```python
from build123d import *

# Parameters (mm, degrees)
SKETCH2_R                   = 9.525
LID_HOLE_DEPTH              = 50.8
SKETCH5_R                   = 12.065
LID_MOUTHPIECE_DEPTH        = 13.97
SKETCH6_R                   = 9.525
LID_HOLE_2_DEPTH            = 59.953263205
LID_HANDLE_DEPTH            = 13.97
SLOT_START                  = -3.302
SKETCH11_R                  = 12.065
SLOT_FOR_COVER_DEPTH        = 3.302
ANGLED_MOUTHPIECE_CUT_DEPTH = 12.7
CUT_EXTRUDE3_START          = -27.94
SKETCH15_R                  = 0.811013261
CUT_EXTRUDE3_DEPTH          = 27.94


with BuildPart() as part:
    # Sketch1 → Lid Shape (revolve)
    with BuildSketch(Plane(origin=(0, 0, 0), x_dir=(1, 0, 0), z_dir=(0, 1, 0))):
        Polygon((0, 50.10238266), (31.75, 50.10238266), (31.75, 25.87078266), (29.21, 25.87078266), (29.21, 40.51388266), (29.21, 41.597899191), (24.13, 41.597899191), (24.13, 40.51388266), (0, 40.51388266), align=None)
    revolve(axis=Axis((0, 0, 0), (0, 0, -1)))

    # Sketch2 → Lid Hole (cut)
    with BuildSketch(Plane.XY.offset(-40.51388266)):
        with Locations((14.478, 0)):
            Circle(SKETCH2_R)
    extrude(amount=-LID_HOLE_DEPTH, mode=Mode.SUBTRACT)

    # Sketch5 → Lid Mouthpiece (add)
    with BuildSketch(Plane(origin=(0, 0, -50.10238266), x_dir=(-1, 0, 0), z_dir=(0, 0, -1))):
        with Locations((-14.478, 0)):
            Circle(SKETCH5_R)
    extrude(amount=LID_MOUTHPIECE_DEPTH)

    # Sketch6 → Lid Hole 2 (cut, through all)
    with BuildSketch(Plane(origin=(0, 0, -64.07238266), x_dir=(-1, 0, 0), z_dir=(0, 0, -1))):
        with Locations(Location((-14.478, 0, 0), (0, 0, 180))):
            Circle(SKETCH6_R)
    extrude(amount=-LID_HOLE_2_DEPTH, mode=Mode.SUBTRACT)

    # Sketch8 → Lid Handle (add, symmetric)
    with BuildSketch(Plane(origin=(0, 0, 0), x_dir=(1, 0, 0), z_dir=(0, 1, 0))):
        Polygon((-31.75, 50.10238266), (-52.891013527, 66.999169477), (-54.31959445, 68.140951412), (-48.565910523, 68.140951412), (-25.996316072, 50.10238266), align=None)
    extrude(amount=LID_HANDLE_DEPTH, both=True)

    # Sketch9 → Handle Hole section 0
    with BuildSketch(Plane(origin=(14.301912302, 0, -17.894344333), x_dir=(-0.7811575478192837, 0, -0.6243339534936118), z_dir=(0.6243339534936119, 0, -0.7811575478192838))):
        with BuildLine():
            Line((55.080337161, 10.795), (76.670337161, 10.795))
            Line((76.670337161, 10.795), (76.670337161, -10.795))
            Line((76.670337161, -10.795), (55.080337161, -10.795))
            Line((55.080337161, -10.795), (55.080337161, 10.795))
        make_face()
    # Sketch10 → Handle Hole section 1
    with BuildSketch(Plane(origin=(12.059167241, 0, -15.088254384), x_dir=(0.7811575478192838, 0, 0.6243339534936119), z_dir=(-0.6243339534936118, 0, 0.7811575478192837))):
        with BuildLine():
            Line((-81.164870789, 11.43), (-59.574870789, 11.43))
            Line((-59.574870789, 11.43), (-59.574870789, -10.16))
            Line((-59.574870789, -10.16), (-81.164870789, -10.16))
            Line((-81.164870789, -10.16), (-81.164870789, 11.43))
        make_face()
    loft(mode=Mode.SUBTRACT)

    # Sketch11 → Slot for Cover (cut)
    with BuildSketch(Plane(origin=(0, 0, -50.10238266), x_dir=(-1, 0, 0), z_dir=(0, 0, -1)).offset(SLOT_START)):
        with BuildLine():
            ThreePointArc((28.511429287, 13.97), (27.373977798, 16.085019102), (26.079920429, 18.108016192))
            Line((26.079920429, 18.108016192), (-26.079920429, 18.108016192))
            ThreePointArc((-26.079920429, 18.108016192), (-30.299339709, 9.48749246), (-31.75, 0))
            ThreePointArc((-31.75, 0), (-30.299339709, -9.48749246), (-26.079920429, -18.108016192))
            Line((-26.079920429, -18.108016192), (26.079920429, -18.108016192))
            ThreePointArc((26.079920429, -18.108016192), (27.373977798, -16.085019102), (28.511429287, -13.97))
            Line((28.511429287, -13.97), (25.996316072, -13.97))
            Line((25.996316072, -13.97), (5.018618521, -13.97))
            Line((5.018618521, -13.97), (5.018618521, 13.97))
            Line((5.018618521, 13.97), (25.996316072, 13.97))
            Line((25.996316072, 13.97), (28.511429287, 13.97))
        make_face()
        with Locations((-14.478, 0)):
            Circle(SKETCH11_R, mode=Mode.SUBTRACT)
    extrude(amount=SLOT_FOR_COVER_DEPTH, mode=Mode.SUBTRACT)

    # Sketch12 → Angled Mouthpiece Cut (cut, symmetric)
    with BuildSketch(Plane(origin=(0, 0, 0), x_dir=(1, 0, 0), z_dir=(0, 1, 0))):
        Polygon((26.628471811, 67.14025983), (26.628471811, 60.995566014), (2.357445469, 57.350666014), (2.357445469, 67.14025983), align=None)
    extrude(amount=ANGLED_MOUTHPIECE_CUT_DEPTH, both=True, mode=Mode.SUBTRACT)

    # Sketch15 → Cut-Extrude3 (cut)
    with BuildSketch(Plane(origin=(0, 13.97, 0), x_dir=(1, 0, 0), z_dir=(0, 1, 0)).offset(CUT_EXTRUDE3_START)):
        with Locations(Location((-33.050089725, 53.387241314, 0), (0, 0, 231.366681908))):
            Circle(SKETCH15_R)
    extrude(amount=CUT_EXTRUDE3_DEPTH, mode=Mode.SUBTRACT)


solid = part.part
```
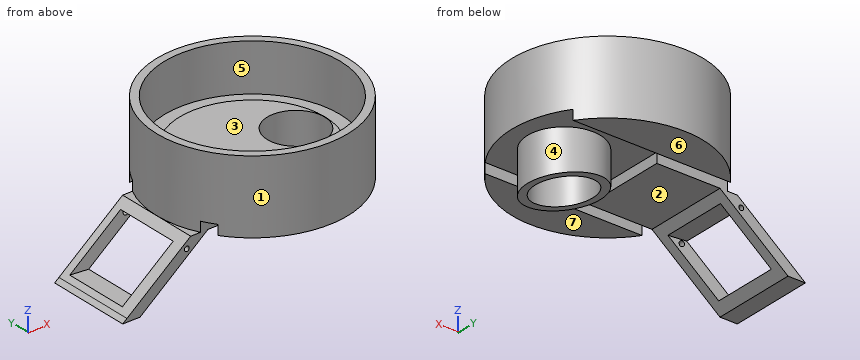
Model file for the job. Use its own axes, mm. Face numbers are marked on the shaded views. A direction names the side the tool comes from. Round coordinates to 2 decimals unless told otherwise and drop trailing zeros. Loops run counter-clockwise (first coordinate to the right, second up) from the corner with the lowest first, then second, coordinate; pieces in that order, holes last. Notation, with made-up numbers: M -26.5,70 L -15.5,70 A22 ccw -15.5,81 Z; hole C -32,-32 d1. An arc over 180 degrees is marked long. Put each result on its own line as item: value. Start each with the question number.
Item 1: 3-axis set-ups, long thin cutter, end or side, ignore diameter. For the marked faces 5, 6 and 7: which of +Z, -Z, +X, -X, +Y, -Y reach the whole face in a straight line?
Item 2: Cut at B-B (x = 0). List the corners of the cut face in (y, z).
Item 3: Cut at C-C (z = -37). List the corners of the cut face in (x, y), then the cut area to 3 significant figures.
Item 4: Mould opens along Y. For the marked faces 1, 2, 3 and 4 say: released by +Y, released by -Y, zero draft, split by the parting line, or undercut.
Item 5: Cut at D-D (y = 16). List the corners of the cut face in (x, z).
Item 6: Drill centre lines: line 1 along X through (y, z) = (0, -44); line 2 along Y through (x, z) = (0, -35.5). Where is each one in solid material? Low to high.
Item 7: Cut at A-A (x = 13.5). List the corners of the cut face in (y, z), then the cut area to 3 significant figures.
Item 8: Drop flat-ended pins along their axis: P1, Ø1.9, axis at x = -33.05, z = -53.39, coming from the -Y side; P2, Ø4, axis at x = 3.5, y = 23, coming from the -Z side; P3, Ø10, axis at x = 9, y = 14, coming from the +Z side; P4, Ø8, axis at y = -2.5, z = -37.5, coming from the +X side. Give the stop position or say it passes through.
Answer block:
1. face 5: +Z
1. face 6: -Z, +X, -X, +Y
1. face 7: -Z, +X, -X, -Y
2. outline: M -31.75,-50.1 L -18.11,-50.1 L -18.11,-46.8 L 18.11,-46.8 L 18.11,-50.1 L 31.75,-50.1 L 31.75,-25.87 L 29.21,-25.87 L 29.21,-41.6 L 24.13,-41.6 L 24.13,-40.51 L -24.13,-40.51 L -24.13,-41.6 L -29.21,-41.6 L -29.21,-25.87 L -31.75,-25.87 Z
3. outline: C 0,0 d63.5; hole C 0,0 d58.42
3. area: 486 mm2
4. face 1: split by the parting line
4. face 2: zero draft
4. face 3: undercut
4. face 4: undercut
5. outline: M -27.42,-46.8 L 27.42,-46.8 L 27.42,-25.87 L 24.44,-25.87 L 24.44,-41.6 L 18.06,-41.6 L 18.06,-40.51 L -18.06,-40.51 L -18.06,-41.6 L -24.44,-41.6 L -24.44,-25.87 L -27.42,-25.87 Z
6. line 1: -31.75 to 4.95, 24 to 31.75
6. line 2: -31.75 to -29.21, 29.21 to 31.75
7. outline: M -28.74,-50.1 L -18.11,-50.1 L -18.11,-46.8 L -12.03,-46.8 L -12.03,-59.02 L -9.47,-59.02 L -9.47,-40.51 L -20,-40.51 L -20,-41.6 L -25.9,-41.6 L -25.9,-25.87 L -28.74,-25.87 Z; M 9.47,-59.02 L 12.03,-59.02 L 12.03,-46.8 L 18.11,-46.8 L 18.11,-50.1 L 28.74,-50.1 L 28.74,-25.87 L 25.9,-25.87 L 25.9,-41.6 L 20,-41.6 L 20,-40.51 L 9.47,-40.51 Z
7. area: 445 mm2
8. P1: y = -13.97
8. P2: z = -50.1
8. P3: z = -40.51
8. P4: x = 31.75
